Work out the finished part from the listing and answer in its coordinate system (mm). A direction names the side the tool comes from. Coordinates: 2 decimals unless noted, no trailing zeros. Order: outer loops, then holes, each group sorted by start corner. A loop starts at its lowest first (then second) coordinate and runs counter-clockwise, first axis right, second up. Notation, with made-up numbers: (24.25, 78.5) -> (38.25, 78.5) arc R16 ccw to (38.25, 93.5) -> close; hole circle Ø2 at (-10.75, -0.5). An arc over 180 degrees is marked (long way). Use one line per item in the form item = value.
from build123d import *

# Parameters (mm, degrees)
F1_DEPTH = 22
F2_T     = 1.5
F3_W     = 9.2
F3_H     = 22
F4_DEPTH = 1.5
F5_R     = 1


with BuildPart() as f1:
    # F0 (on Top) → F1 (new body)
    with BuildSketch(Plane.XY):
        with BuildLine():
            Line((-4.6, -5.9236812878), (-4.6, -22))
            Line((-4.6, -22), (4.6, -22))
            Line((4.6, -22), (4.6, -5.9236812878))
            ThreePointArc((4.6, -5.9236812878), (0, 7.5), (-4.6, -5.9236812878))
        make_face()
    extrude(amount=F1_DEPTH)

    # F2
    f2_openings = [f1.faces().sort_by_distance(p)[0] for p in [
        (0, -6.355052, 22),
    ]]
    offset(amount=F2_T, openings=f2_openings, kind=Kind.INTERSECTION)

    # F3 (on face) → F4 (cut, through all)
    with BuildSketch(Plane.XZ.offset(23.5)):
        with Locations((0, 11)):
            Rectangle(F3_W, F3_H)
    extrude(amount=-F4_DEPTH, mode=Mode.SUBTRACT)

    # F5
    f5_edges = [f1.edges().sort_by_distance(p)[0] for p in [
        (6.1, -23.5, 10.25),
        (-6.1, -23.5, 10.25),
        (0, -23.5, -1.5),
        (-6.1, -15.058701, -1.5),
        (6.1, -15.058701, -1.5),
        (0, 9, -1.5),
    ]]
    fillet(f5_edges, radius=F5_R)


solid = f1.part
(1) Section A-A on z = 18.75 is taken. Write down the section's boundary in (x, y), plus the area to 3 significant figures.
Data:
outline = (-6.1, -22.5) arc R1 ccw to (-5.1, -23.5) -> (-4.6, -23.5) -> (-4.6, -5.92) arc R7.5 cw (long way) to (4.6, -5.92) -> (4.6, -23.5) -> (5.1, -23.5) arc R1 ccw to (6.1, -22.5) -> (6.1, -6.62) arc R9 ccw (long way) to (-6.1, -6.62) -> close
area = 112 mm²
(2) Straight lines are drawn through the part: line 1 along X through (y, z) = (0, 9); line 2 along X through (y, z) = (-21.5, 1); line 3 along Z through (x, y) = (-1, 3). For each, find the intervals that lie inside material, in ascending order.
Data:
line_1 = -9 to -7.5, 7.5 to 9
line_2 = -6.1 to -4.6, 4.6 to 6.1
line_3 = -1.5 to 0
(3) The mould has two halves that part along X. Classify faces 5 (the flat face through (0, -7, -1.5)), 6 (the flat face through (6.1, -15, 11)), 7 (the flat face through (-4.6, -15, 11)), 8 (the cylindrical face through (0.26, 7.495, 10.846)): released by +X, released by -X, zero draft, split by the parting line, or undercut.
Data:
face_5 = zero draft
face_6 = released by +X
face_7 = undercut
face_8 = undercut
(4) Section C-C on y = -18.5 is taken. Write down the section's boundary in (x, z), plus the area to 3 significant figures.
Data:
outline = (-6.1, -0.5) arc R1 ccw to (-5.1, -1.5) -> (5.1, -1.5) arc R1 ccw to (6.1, -0.5) -> (6.1, 22) -> (4.6, 22) -> (4.6, 0) -> (-4.6, 0) -> (-4.6, 22) -> (-6.1, 22) -> close
area = 83.9 mm²
(5) Section B-B on x = 0 is taken. Write down the section's boundary in (y, z).
Data:
outline = (-23.5, -0.5) arc R1 ccw to (-22.5, -1.5) -> (8, -1.5) arc R1 ccw to (9, -0.5) -> (9, 22) -> (7.5, 22) -> (7.5, 0) -> (-23.5, 0) -> close
(6) Each of these flat-tipped pins is pushed along its axis until it touches: P1, Ø4, axis at x = -3.5, z = 5.5, coming from the +Y side; P2, Ø6, axis at y = -16.5, z = 6, coming from the +X side; P3, Ø9, axis at y = -19, z = 6.5, coming from the -X side. Where does it stop, or does it pass through?
Data:
P1 = 8.87
P2 = 6.1
P3 = -6.1
(7) Which of the six approach directions +Z, -Z, +X, -X, +Y, -Y give full straight-line access (tool end or side, diameter ignored) to faces 1 (the flat face through (-6.1, -14, 11)), 2 (the flat face through (4.6, -15, 11)), 3 (the flat face through (0, -8, 0)), 4 (the cylindrical face through (5.799, -14.217, -1.215))?
Data:
face_1 = +Z, -Z, -X, -Y
face_2 = +Z, -Y
face_3 = +Z
face_4 = -Z, +X, -Y
